The listing builds one solid part. Answer for the finished solid, in the listing's coordinates (mm). A direction names the side the tool comes from. Coordinates: 2 decimals unless noted, no trailing zeros. Loops run counter-clockwise (first coordinate to the right, second up) from the corner with the lowest first, then second, coordinate; pieces in that order, holes last. Notation, with made-up numbers: M 31,-5.5 L 66,-5.5 A24 ccw 66,5.5 Z; hole C 53.25,38 d6. An arc over 180 degrees is marked long. Return JSON: item names as keys, results as strings. Group by question number.
1. Section B-B (y = 10) is taken. Write down the section's boundary in (x, z).
2. Section A-A (z = 22.25) is taken. Write down the section's boundary in (x, y), then the cut area to 3 significant figures.
3. Straight lines are drawn through the part: L1, parallel to Y at x = 0, z = 11; L2, parallel to X at y = 10, z = 5.5; L3, parallel to Y at x = -4.75, z = 23.75. For each, find the intervals that lie inside material, in ascending order. Write a range as from..to.
4. Which of the six approach directions +Z, -Z, +X, -X, +Y, -Y give full straight-line access (tool end or side, diameter ignored) to faces 4 (the face through (-7.5, -0.2, 13.9)), 5 (the face through (7.5, -0.2, 13.9)), 6 (the face through (0, 15, 25))?
5. The mould has two halves that part along X. Classify faces 1 (the face through (0, -20, 12)), 2 (the face through (5, 0, 18)), 3 (the face through (-0.117, -7.353, 12.325)): pulls with the +X half, pulls with the -X half, needs draft (parallel to the pull), parting line crosses it, or undercut.
6. Section C-C (y = 0) is taken. Write down the section's boundary in (x, z), then the cut area to 3 significant figures.
7. Given P1, Ø12, axis at x = 6.5, y = -5.5, coming from the +Z side; P2, Ø3.5, axis at y = 2.5, z = 17, coming from the +X side, each flat-ended and moving along its own axis, determine where each tip first touches the part or whether it passes through.
8. Section D-D (z = 15.5) is taken. Write down the section's boundary in (x, y).
Autodesk Inventor part; units mm, degrees
ref_plane "YZ Plane" through (0, 0, 0) normal (1, 0, 0) x (0, 1, 0)
ref_plane "XZ Plane" through (0, 0, 0) normal (0, 1, 0) x (-1, 0, 0)
ref_plane "XY Plane" through (0, 0, 0) normal (0, 0, 1) x (1, 0, 0)
sketch "スケッチ1" plane through (0, 0, 0) normal (0, 0, 1) x (1, 0, 0)
  line L0 (-10, -20) -> (10, -20)
  line L1 (10, -20) -> (10, 20)
  line L2 (10, 20) -> (-10, 20)
  line L3 (-10, 20) -> (-10, -20)
  line L4 (-10, -20) -> (10, 20) construction
  line L5 (10, -20) -> (-10, 20) construction
  point P0 (0, 0)
  dimension "d0" = 20
  dimension "d1" = 40
extrude "押し出し1" add sketch "スケッチ1" along normal blind 25
sketch "スケッチ2" plane through (10, -20, 0) normal (1, 0, 0) x (0, 0, -1)
  circle A0 centre (-25, 20) radius 11.1
  line L0 (0, 40) -> (-25, 40)
  dimension "d4" = 22.2
  dimension "d7" = 20
extrude "押し出し2" cut sketch "スケッチ2" against normal through all
sketch "スケッチ7" plane through (0, 0, 0) normal (1, 0, 0) x (0, 1, 0)
  arc A0 (-11.1, 25) -> (11.1, 25) centre (0, 25) ccw
  line L0 (20, 25) -> (11.1, 25)
  line L1 (20, 0) -> (20, 25)
  line L2 (20, 0) -> (-20, 0)
  line L3 (-20, 0) -> (-20, 25)
  line L4 (-11.1, 25) -> (-20, 25)
  circle A1 centre (0, 25) radius 6
  arc A2 (-11.1, 25) -> (11.1, 25) centre (0, 25) ccw
  line L5 (11.1, 25) -> (-11.1, 25)
  point P0 (0, 0)
  point P1 (-6, 25)
  point P2 (6, 25)
  dimension "d27" = 12
extrude "押し出し5" add sketch "スケッチ7" along normal mid plane 10 contours L5 A1 A0
sketch "スケッチ5" plane through (0, 0, 25) normal (0, 0, 1) x (1, 0, 0)
  line L0 (10, 20) -> (-10, 20)
  line L1 (-10, -20) -> (10, -20)
  point P0 (0, 0)
  point P1 (0, 10)
  point P2 (0, -10)
  dimension "d18" = 10
  dimension "d19" = 10
hole "穴1" at (0, 10, 25) at (0, -10, 25) direction (0, 0, -1) diameter 5.3 depth 58
properties part number "Print_Parts_A2" material "PC/ABS プラスチック"
Worked out:
{
 "1": {"outline": "M -10,0 L -2.65,0 L -2.65,25 L -5,25 L -5,20.18 L -10,20.18 Z; M 2.65,0 L 10,0 L 10,20.18 L 5,20.18 L 5,25 L 2.65,25 Z"},
 "2": {"outline": "M -10,-20 L 10,-20 L 10,-10.75 L 5,-10.75 L 5,-5.33 L -5,-5.33 L -5,-10.75 L -10,-10.75 Z; M -10,10.75 L -5,10.75 L -5,5.33 L 5,5.33 L 5,10.75 L 10,10.75 L 10,20 L -10,20 Z; hole C 0,-10 d5.3; hole C 0,10 d5.3", "area": "434 mm^2"},
 "3": {"L1": "-20..-12.65, -7.35..7.35, 12.65..20", "L2": "-10..-2.65, 2.65..10", "L3": "-20..-5.87, 5.87..20"},
 "4": {"face 4": "+Z, -X", "face 5": "+Z, +X", "face 6": "+Z, +X, -X, +Y, -Y"},
 "5": {"face 1": "needs draft", "face 2": "pulls with the +X half", "face 3": "undercut"},
 "6": {"outline": "M -10,0 L 10,0 L 10,13.9 L 5,13.9 L 5,19 L -5,19 L -5,13.9 L -10,13.9 Z", "area": "329 mm^2"},
 "7": {"P1": "z = 25", "P2": "x = 5"},
 "8": {"outline": "M -10,-20 L 10,-20 L 10,-5.74 L 5,-5.74 L 5,5.74 L 10,5.74 L 10,20 L -10,20 L -10,5.74 L -5,5.74 L -5,-5.74 L -10,-5.74 Z; hole C 0,-10 d5.3; hole C 0,10 d5.3"}
}
